Here's how the part is built. I have some questions about the finished solid (model axes, mm). Face numbers are marked on the shaded views. A direction names the side the tool comes from. Give positions to 0.01 mm unless a question says otherwise; leave off trailing zeros. Write each loop counter-clockwise with the first axis right and the second up, starting at its lowest first coordinate (ties: lowest second). Pieces come first, ordered by that corner, then holes. Notation, with made-up numbers: (7.5, 79.5) - (66.5, 79.5) arc R20 cw to (66.5, 117.5) - close; hole circle Ø6 at (64, -30). An arc over 180 degrees is marked (long way). Use a Markdown table: item, result.
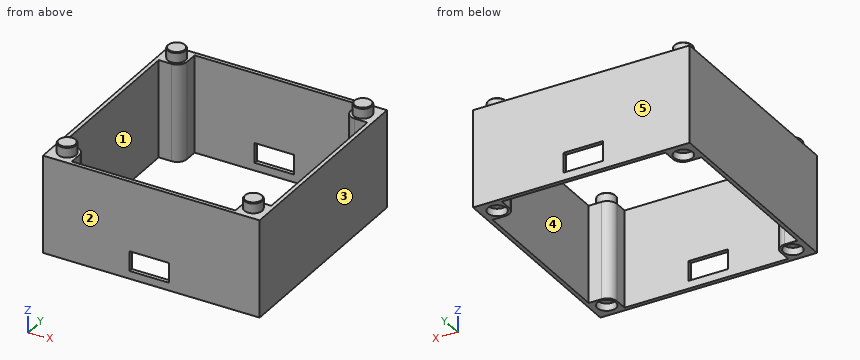
```python
from build123d import *

# Parameters (mm, degrees)
SKICA1_W                 = 5.8
SKICA1_H                 = 5.8
SKICA1_W_2               = 1
SKICA1_H_2               = 42
SKICA1_W_3               = 42
SKICA1_H_3               = 1
P_IDAT_VYSUNUT_M2_DEPTH  = 25
ZAOBLIT1_R               = 2.5
SKICA2_R                 = 2.4
ODEBRAT_VYSUNUT_M1_DEPTH = 1.9
SKICA3_R                 = 2.3
P_IDAT_VYSUNUT_M3_DEPTH  = 2.7
ZKOSEN_1_SIZE            = 0.2
SKICA4_W                 = 10.16
SKICA4_H                 = 5.08
ODEBRAT_VYSUNUT_M2_DEPTH = 68.7


with BuildPart() as part:
    # Skica1 → Přidat vysunutím2 (new body)
    with BuildSketch(Plane.XY):
        Polygon((-27.8, 27.8), (-27.8, 21), (-26.8, 21), (-26.8, 26.8), (-21, 26.8), (-21, 27.8), align=None)
        with Locations((-23.9, 23.9)):
            Rectangle(SKICA1_W, SKICA1_H)
        Polygon((26.8, 21), (27.8, 21), (27.8, 27.8), (21, 27.8), (21, 26.8), (26.8, 26.8), align=None)
        with Locations((23.9, 23.9)):
            Rectangle(SKICA1_W, SKICA1_H)
        Polygon((21, -26.8), (21, -27.8), (27.8, -27.8), (27.8, -21), (26.8, -21), (26.8, -26.8), align=None)
        with Locations((23.9, -23.9)):
            Rectangle(SKICA1_W, SKICA1_H)
        with Locations((-23.9, -23.9)):
            Rectangle(SKICA1_W, SKICA1_H)
        Polygon((-27.8, -27.8), (-21, -27.8), (-21, -26.8), (-26.8, -26.8), (-26.8, -21), (-27.8, -21), align=None)
        with Locations((-27.3, 0)):
            Rectangle(SKICA1_W_2, SKICA1_H_2)
        with Locations((0, -27.3)):
            Rectangle(SKICA1_W_3, SKICA1_H_3)
        with Locations((27.3, 0)):
            Rectangle(SKICA1_W_2, SKICA1_H_2)
        with Locations((0, 27.3)):
            Rectangle(SKICA1_W_3, SKICA1_H_3)
    extrude(amount=P_IDAT_VYSUNUT_M2_DEPTH)

    # Zaoblit1
    zaoblit1_edges = [part.edges().sort_by_distance(p)[0] for p in [
        (21, -21, 12.5),
        (21, 21, 12.5),
        (-21, 21, 12.5),
        (-21, -21, 12.5),
    ]]
    fillet(zaoblit1_edges, radius=ZAOBLIT1_R)

    # Skica2 → Odebrat vysunutím1 (cut)
    with BuildSketch(Plane(origin=(0, 0, 0), x_dir=(-1, 0, 0), z_dir=(0, 0, -1))):
        with Locations((-23.9, 23.9)):
            Circle(SKICA2_R)
        with Locations((23.9, 23.9)):
            Circle(SKICA2_R)
        with Locations((23.9, -23.9)):
            Circle(SKICA2_R)
        with Locations((-23.9, -23.9)):
            Circle(SKICA2_R)
    extrude(amount=-ODEBRAT_VYSUNUT_M1_DEPTH, mode=Mode.SUBTRACT)

    # Skica3 → Přidat vysunutím3 (add)
    with BuildSketch(Plane.XY.offset(25)):
        with Locations((-23.9, 23.9)):
            Circle(SKICA3_R)
        with Locations((23.9, 23.9)):
            Circle(SKICA3_R)
        with Locations((23.9, -23.9)):
            Circle(SKICA3_R)
        with Locations((-23.9, -23.9)):
            Circle(SKICA3_R)
    extrude(amount=P_IDAT_VYSUNUT_M3_DEPTH)

    # Zkosení1
    zkosen_1_edges = [part.edges().sort_by_distance(p)[0] for p in [
        (-26.2, 23.9, 27.7),
        (21.6, 23.9, 27.7),
        (21.6, -23.9, 27.7),
        (-26.2, -23.9, 27.7),
    ]]
    chamfer(zkosen_1_edges, length=ZKOSEN_1_SIZE)

    # Skica4 → Odebrat vysunutím2 (cut)
    with BuildSketch(Plane(origin=(0, -27.8, 0), x_dir=(-1, 0, 0), z_dir=(0, -1, 0))):
        with Locations((0.5, -4.54)):
            Rectangle(SKICA4_W, SKICA4_H)
    extrude(amount=-ODEBRAT_VYSUNUT_M2_DEPTH, mode=Mode.SUBTRACT)


solid = part.part
```
Item 1: Will these pins go through, and if not, where does the flat tip stop? pin 1 Ø1.4 at (x, y) = (-24.5, 24) entering from -Z; pin 2 Ø0.5 at (x, y) = (-1, 27.5) entering from +Z; pin 3 Ø10 at (x, y) = (1, -19.5) entering from +Z.
Values:
| item | result |
|---|---|
| pin 1 | stops at z = 1.9 |
| pin 2 | stops at z = 25 |
| pin 3 | passes through |
Item 2: If we section it at B-B, the plane z = 22: Write out the boundary of the cut face in (x, y), plus the area to 3 significant figures.
Values:
| item | result |
|---|---|
| outline | (-27.8, -27.8) - (27.8, -27.8) - (27.8, 27.8) - (-27.8, 27.8) - close; hole (-26.8, -21) - (-23.5, -21) arc R2.5 cw to (-21, -23.5) - (-21, -26.8) - (21, -26.8) - (21, -23.5) arc R2.5 cw to (23.5, -21) - (26.8, -21) - (26.8, 21) - (23.5, 21) arc R2.5 cw to (21, 23.5) - (21, 26.8) - (-21, 26.8) - (-21, 23.5) arc R2.5 cw to (-23.5, 21) - (-26.8, 21) - close |
| area | 348 mm2 |
Item 3: If we section it at A-A, the plane y = 13.5: Write out the boundary of the cut face in (x, z), plus the area to 3 significant figures.
Values:
| item | result |
|---|---|
| outline | (-27.8, 0) - (-26.8, 0) - (-26.8, 25) - (-27.8, 25) - close; (26.8, 0) - (27.8, 0) - (27.8, 25) - (26.8, 25) - close |
| area | 50.0 mm2 |
Item 4: For the marked faces 1 and 2, which set-ups out of +Z, -Z, +X, -X, +Y, -Y let a thin tool reach every point of the face, with its end or its side?
Values:
| item | result |
|---|---|
| face 1 | +Z, -Z |
| face 2 | +Z, -Z, +X, -X, -Y |
Item 5: I need wall thicknesses on line 1 along Y through (x, z) = (-23.9, 1.15); line 2 along X through (y, z) = (-8, 9.5). Which ranges of each line are inside material? Lowest first, please. Write a range as [from, to].
Values:
| item | result |
|---|---|
| line 1 | y = [-27.8, -26.3], [-21.5, -21], [21, 21.5], [26.3, 27.8] |
| line 2 | x = [-27.8, -26.8], [26.8, 27.8] |
Item 6: Thinking about a two-plate mould opening in X: for the marked faces 3, 4 and 5, which applies, +X half, -X half, draft (parallel to the pull), parting line (faces both ways), or undercut?
Values:
| item | result |
|---|---|
| face 3 | +X half |
| face 4 | undercut |
| face 5 | draft |
